from build123d import *

# Parameters (mm, degrees)
SKETCH2_W           = 20
SKETCH2_H           = 14
BOSS_EXTRUDE2_DEPTH = 2
BOSS_EXTRUDE3_DEPTH = 5
SKETCH4_R           = 2
CUT_EXTRUDE1_DEPTH  = 21


with BuildPart() as part:
    # Sketch2 → Boss-Extrude2 (new body)
    with BuildSketch(Plane(origin=(0, 0, 0), x_dir=(1, 0, 0), z_dir=(0, 1, 0))):
        Rectangle(SKETCH2_W, SKETCH2_H)
    extrude(amount=BOSS_EXTRUDE2_DEPTH)

    # Sketch3 → Boss-Extrude3 (add)
    with BuildSketch(Plane(origin=(10, 0, 0), x_dir=(0, 0, -1), z_dir=(1, 0, 0))):
        with BuildLine():
            Line((12, 2), (7, 2))
            Line((7, 2), (7, 0))
            Line((7, 0), (8, 0))
            ThreePointArc((8, 0), (10.618033989, -0.236067977), (12, 2))
        make_face()
        with BuildLine():
            ThreePointArc((12, 2), (9.5, 4.5), (7, 2))
            Line((7, 2), (12, 2))
        make_face()
    boss_extrude3 = extrude(amount=-BOSS_EXTRUDE3_DEPTH)

    # Mirror1: Boss-Extrude3 across plane
    add(boss_extrude3.mirror(Plane.ZY.offset(-2.5)))

    # Sketch4 → Cut-Extrude1 (cut, through all)
    with BuildSketch(Plane(origin=(10, 0, 0), x_dir=(0, 0, -1), z_dir=(1, 0, 0))):
        with Locations((9.5, 2)):
            Circle(SKETCH4_R)
    extrude(amount=-CUT_EXTRUDE1_DEPTH, mode=Mode.SUBTRACT)


solid = part.part
Verification items for the finished model (mm, model axes). A direction names the side the tool comes from. Give positions to 0.01 mm unless a question says otherwise; leave off trailing zeros. Write each loop counter-clockwise with the first axis right and the second up, starting at its lowest first coordinate (ties: lowest second). Pieces come first, ordered by that corner, then holes.
(1) Cross-section at B-B (y = 3.25). Enter the section's corners in (x, z).
(2) Cross-section at C-C (x = -0.75). Enter the section's corners in (y, z).
(3) Access from +Z, -Z, +X, -X, +Y, -Y to the whole of each face (thin tool, end or side, straight path). Record for faces 4 (the face through (0, 2, 0)), 5 (the face through (2, 1, -7)), 6 (the face through (0, 1, 7)), 7 (the face through (0, 0, 0)), 8 (the face through (7.5, 0.8, -7.9)).
(4) Mould release check, pull along Z, two halves, no side actions. Record for faces 1 (the face through (-10, 1, 0)), 2 (the face through (-2.5, 0.8, -7.9)), 3 (the face through (-8, 1, -7)): +Z half, -Z half, draft (parallel to the pull), parting line (faces both ways), or undercut.
(5) Gauge pin test, flat ends, axial feed: pin 1 (0.6 mm diameter, centred on x = 3, y = 1, fed in from -Z); pin 2 (1 mm diameter, centred on x = 6.5, z = 3.5, fed in from +Y); pin 3 (2.5 mm diameter, centred on y = 1.5, z = -8.5, fed in from -X); pin 4 (2.5 mm diameter, centred on y = 2, z = -9.5, fed in from -X). Record the tip position at first contact, or that the pin passes through.
(6) Cross-section at A-A (z = -9.5). Enter the section's corners in (x, y), plus the area to 4 significant figures.
(7) Material ranges on line 1 (X direction, y = 0.8, z = -7.25); line 2 (Y direction, x = 6.1, z = -9.5); line 3 (Z direction, x = -3.5, y = 1.9), recorded low to high.
(8) Cross-section at D-D (y = 1.35). Enter the section's corners in (x, z), plus the area to 3 significant figures.
Worked out:
1. outline: (-5, -11.67) - (0, -11.67) - (0, -11.06) - (-5, -11.06) - close; (-5, -7.94) - (0, -7.94) - (0, -7.33) - (-5, -7.33) - close; (5, -11.67) - (10, -11.67) - (10, -11.06) - (5, -11.06) - close; (5, -7.94) - (10, -7.94) - (10, -7.33) - (5, -7.33) - close
2. outline: (0, -8) arc R2.5 ccw (long way) to (2, -7) - (2, 7) - (0, 7) - close; hole circle Ø4 at (2, -9.5)
3. face 4: +Z, +X, -X, +Y
3. face 5: -Z, +Y, -Y
3. face 6: +Z, +X, -X, +Y, -Y
3. face 7: +Z, +X, -X, -Y
3. face 8: +X, -X
4. face 1: draft
4. face 2: undercut
4. face 3: -Z half
5. pin 1: stops at z = -7
5. pin 2: stops at y = 2
5. pin 3: stops at x = -5
5. pin 4: passes through
6. outline: (-5, -0.5) - (0, -0.5) - (0, 0) - (-5, 0) - close; (-5, 4) - (0, 4) - (0, 4.5) - (-5, 4.5) - close; (5, -0.5) - (10, -0.5) - (10, 0) - (5, 0) - close; (5, 4) - (10, 4) - (10, 4.5) - (5, 4.5) - close
6. area: 10.00 mm2
7. line 1: x = -5 to 0, 5 to 10
7. line 2: y = -0.5 to 0, 4 to 4.5
7. line 3: z = -12 to -11.5, -7.5 to 7
8. outline: (-10, -7) - (-5, -7) - (-5, -7.61) - (0, -7.61) - (0, -7) - (5, -7) - (5, -7.61) - (10, -7.61) - (10, 7) - (-10, 7) - close; (-5, -11.91) - (0, -11.91) - (0, -11.39) - (-5, -11.39) - close; (5, -11.91) - (10, -11.91) - (10, -11.39) - (5, -11.39) - close
8. area: 291 mm2
